Part model, mm, in its own coordinate system. Face numbers are marked on the shaded views. A direction names the side the tool comes from. Round coordinates to 2 decimals unless told otherwise and drop trailing zeros. Loops run counter-clockwise (first coordinate to the right, second up) from the corner with the lowest first, then second, coordinate; pieces in that order, holes last. Notation, with made-up numbers: (-35.5, 64) -> (-30.5, 64) arc R10 cw to (-30.5, 76) -> close; hole circle Ø5 at (-13.75, -8.75). An arc over 180 degrees is marked (long way). Answer as CSV lines item,"result".
from build123d import *

# Parameters (mm, degrees)
F0_R     = 6.35
F1_DEPTH = 2.5
F2_R     = 4
F3_DEPTH = 0.9
F4_R     = 2
F5_DEPTH = 3.401


with BuildPart() as f1:
    # F0 (on Top) → F1 (new body)
    with BuildSketch(Plane.XY):
        Circle(F0_R)
    extrude(amount=F1_DEPTH)

    # F2 (on face) → F3 (join)
    with BuildSketch(Plane.XY.offset(2.5)):
        Circle(F2_R)
    extrude(amount=F3_DEPTH)

    # F4 (on face) → F5 (cut, through all)
    with BuildSketch(Plane.XY.offset(3.4)):
        Circle(F4_R)
    extrude(amount=-F5_DEPTH, mode=Mode.SUBTRACT)


solid = f1.part
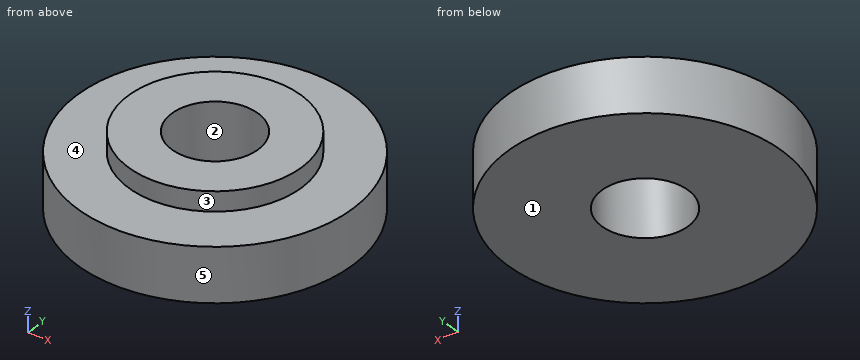
Q1. Saw through at C-C, the plane z = 1.5. Write the cut outline in (x, y).
Geometry results:
outline,"circle Ø12.7 at (0, 0); hole circle Ø4 at (0, 0)"
Q2. Saw through at A-A, the plane y = 0. Write the cut outline in (x, z).
Geometry results:
outline,"(-6.35, 0) -> (-2, 0) -> (-2, 3.4) -> (-4, 3.4) -> (-4, 2.5) -> (-6.35, 2.5) -> close; (2, 0) -> (6.35, 0) -> (6.35, 2.5) -> (4, 2.5) -> (4, 3.4) -> (2, 3.4) -> close"
Q3. Drop flat-ended pins along their axis: P1, Ø1.5, axis at y = 2, z = 1.5, coming from the +X side; P2, Ø2, axis at y = 3.5, z = 1, coming from the -X side; P3, Ø1, axis at y = -2, z = 1, coming from the -X side. Give the stop position or say it passes through.
Geometry results:
P1,"x = 6.23"
P2,"x = -5.84"
P3,"x = -6.17"
Q4. Saw through at D-D, the plane x = 3.75. Write the cut outline in (y, z).
Geometry results:
outline,"(-5.12, 0) -> (5.12, 0) -> (5.12, 2.5) -> (1.39, 2.5) -> (1.39, 3.4) -> (-1.39, 3.4) -> (-1.39, 2.5) -> (-5.12, 2.5) -> close"
Q5. Which spindle directions (+Z, -Z, +X, -X, +Y, -Y) get a long thin tool onto all of the face, cutting with end or side? Do the marked faces 4 and 5. Say none if no direction does.
Geometry results:
face 4,"+Z"
face 5,"+Z, -Z"
Q6. Two-plate mould, pull along X, no slides. Class the marked faces 1, 2 and 3: pulls with the +X half, pulls with the -X half, needs draft (parallel to the pull), parting line crosses it, or undercut.
Geometry results:
face 1,"needs draft"
face 2,"undercut"
face 3,"parting line crosses it"
Q7. Drill centre lines: line 1 along Z through (x, y) = (4.25, 2.5); line 2 along Y through (x, z) = (0, 1.3); line 3 along X through (y, z) = (-0.25, 1.2). Where is each one in solid material? Low to high.
Geometry results:
line 1,"0 to 2.5"
line 2,"-6.35 to -2, 2 to 6.35"
line 3,"-6.35 to -1.98, 1.98 to 6.35"
